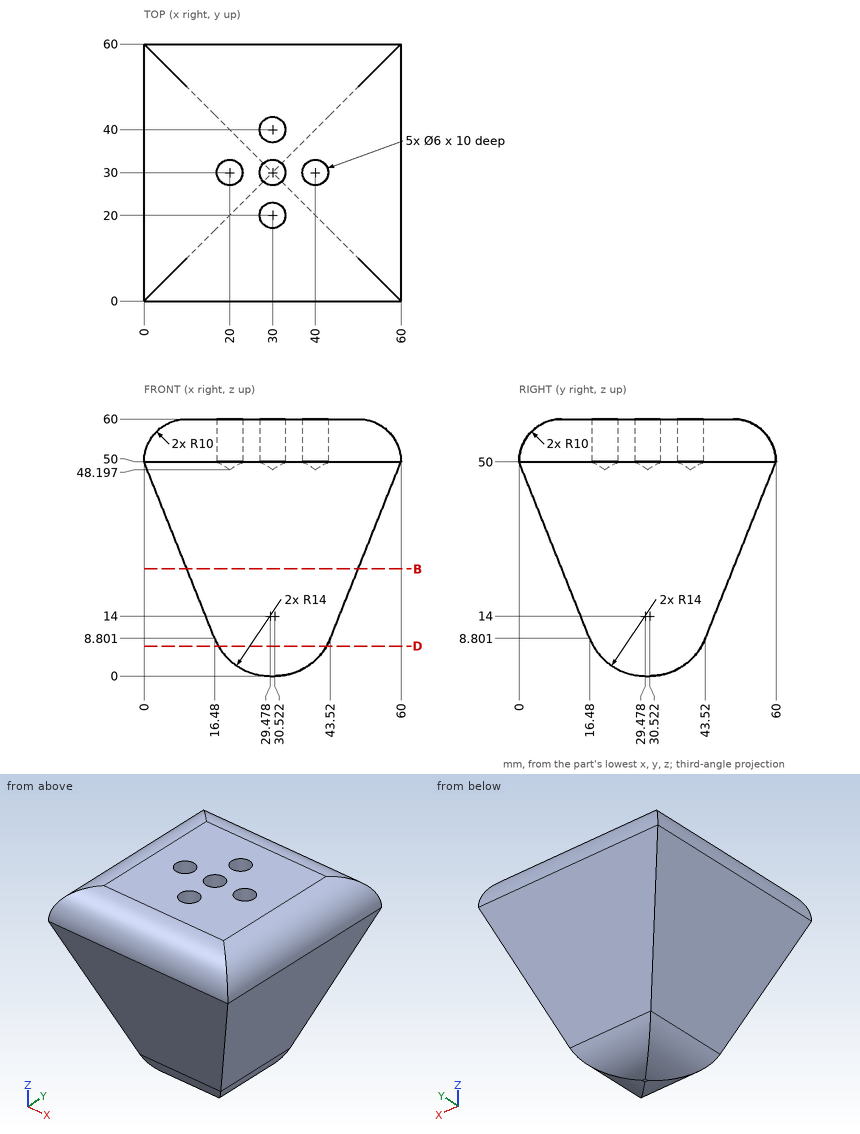
Check sheet for the drawn part. Datum: minimum x, y, z corner. Units: mm. Give positions to 0.01 mm unless a question says otherwise; leave off trailing zeros. Order: outer loops, then holes, each group sorted by start corner. A loop starts at its lowest first (then second) coordinate and runs counter-clockwise, first axis right, second up. Notation, with made-up numbers: (48.25, 32) - (80.25, 32) arc R15 cw to (80.25, 47) - close; hole circle Ø3 at (-35, 53). An arc over 180 degrees is marked (long way). Answer as a JSON object with one key per item and string values.
(1) Cross-section at D-D (z = 7). Record the cut outline in (x, y) (1 decimal).
Report:
{"outline": "(17.4, 17.4) - (42.6, 17.4) - (42.6, 42.6) - (17.4, 42.6) - close"}
(2) Material ranges on line 1 (Y direction, x = 30, z = 55); line 2 (Y direction, x = 31, z = 58.5) (1 decimal); line 3 (X direction, y = 40, z = 56.75), recorded low to high.
Report:
{"line 1": "1.34 to 17, 23 to 27, 33 to 37, 43 to 58.66", "line 2": "4.7 to 17.2, 22.8 to 27.2, 32.8 to 37.2, 42.8 to 55.3", "line 3": "2.62 to 27, 33 to 57.38"}
(3) Depth check by flat-ended pin: pin 1 Ø8 at (y, z) = (12.5, 13) entering from -X; pin 2 Ø5.5 at (x, y) = (30, 40) entering from +Z; pin 3 Ø8 at (x, z) = (52, 40.5) entering from +Y; pin 4 Ø2 at (y, z) = (9, 22) entering from -X. Enter the tip coordinate at first touch or a pass-through.
Report:
{"pin 1": "x = 13.23", "pin 2": "z = 49.85", "pin 3": "y = 57.8", "pin 4": "through"}
(4) Cross-section at B-B (z = 25). Record the cut outline in (x, y).
Report:
{"outline": "(10, 10) - (50, 10) - (50, 50) - (10, 50) - close"}
